Geometry: final body of the model. Coordinates: model frame, mm. A direction names the side the tool comes from. Round coordinates to 2 decimals unless told otherwise and drop trailing zeros. Loops run counter-clockwise (first coordinate to the right, second up) from the corner with the lowest first, then second, coordinate; pieces in that order, holes last. Notation, with made-up numbers: (0, -23.5) - (46, -23.5) arc R3 cw to (46, -18.5) - close; hole circle Ø9 at (61.25, -8.5). An arc over 180 degrees is marked (long way). Answer as a JSON object with one key per item and string values. Group by question number.
Item 1: Reachability of faces 1 (the face through (0, 0, -0.4)), 2 (the face through (4.91, 1.55, 0.74)) from +Z, -Z, +X, -X, +Y, -Y: full face, straight path, thin tool, end or side. Return the list, or none.
Item 2: First-contact query: pin 1 (2 mm diameter, centred on y = 2, z = 13, fed in from +X); pin 2 (10 mm diameter, centred on x = -5, y = -2, fed in from +Z); pin 3 (1 mm diameter, centred on y = -4, z = 12, fed in from -X). Flat tips, straight axial feed; report the tip coordinate or a pass-through.
Item 3: Section B-B (y = 11). Return the cut outline in (x, z), plus the area to 3 significant figures.
Item 4: Section A-A (x = 0). Return the cut outline in (y, z), plus the area to 3 significant figures.
Item 5: Section D-D (y = -0.5). Return the cut outline in (x, z), plus the area to 3 significant figures.
Item 6: Draft query along Y for faces 3 (the face through (-1.116, 5.972, 0.537)), 4 (the face through (5.4, -16.4, 16)). Return one class per face: released by +Y, released by -Y, zero draft, split by the parting line, or undercut.
Item 7: Line query: line 1 (Y direction, x = 0, z = 0.5); line 2 (Z direction, x = 8.5, y = 0); line 3 (X direction, y = -1, z = 13.25). Output: solid intervals per line, ascending.
Item 8: Section C-C (x = 9.5). Return the cut outline in (y, z), plus the area to 3 significant figures.
```python
from build123d import *

# Parameters (mm, degrees)
F2_R     = 18.5
F2_R_2   = 17
F2_R_3   = 5.15
F3_DEPTH = 0.4
F4_DEPTH = 1.5
F5_DEPTH = 16


with BuildPart() as f3:
    # F2 (on Top) → F3 (new body)
    with BuildSketch(Plane.XY):
        Circle(F2_R)
        Circle(F2_R_2, mode=Mode.SUBTRACT)
        Circle(F2_R_2)
        with Locations((0, -11)):
            Circle(F2_R_3, mode=Mode.SUBTRACT)
        Circle(F2_R_3, mode=Mode.SUBTRACT)
        with Locations((0, 11)):
            Circle(F2_R_3, mode=Mode.SUBTRACT)
        Circle(F2_R_3)
        with Locations((0, -11)):
            Circle(F2_R_3)
    extrude(amount=-F3_DEPTH)

    # F2 (on Top) → F4 (join)
    with BuildSketch(Plane.XY):
        Circle(F2_R_2)
        with Locations((0, -11)):
            Circle(F2_R_3, mode=Mode.SUBTRACT)
        Circle(F2_R_3, mode=Mode.SUBTRACT)
        with Locations((0, 11)):
            Circle(F2_R_3, mode=Mode.SUBTRACT)
    extrude(amount=F4_DEPTH)

    # F2 (on Top) → F5 (join)
    with BuildSketch(Plane.XY):
        Circle(F2_R)
        Circle(F2_R_2, mode=Mode.SUBTRACT)
    extrude(amount=F5_DEPTH)


solid = f3.part
```
Values:
{
 "1": {"face 1": "-Z, +X, -X, +Y, -Y", "face 2": "+Z"},
 "2": {"pin 1": "stops at x = 18.47", "pin 2": "stops at z = 1.5", "pin 3": "stops at x = -18.17"},
 "3": {"outline": "(-14.87, -0.4) - (-5.15, -0.4) - (-5.15, 1.5) - (-12.96, 1.5) - (-12.96, 16) - (-14.87, 16) - close; (5.15, -0.4) - (14.87, -0.4) - (14.87, 16) - (12.96, 16) - (12.96, 1.5) - (5.15, 1.5) - close", "area": "92.4 mm^2"},
 "4": {"outline": "(-18.5, -0.4) - (5.85, -0.4) - (5.85, 1.5) - (5.15, 1.5) - (5.15, 0) - (-5.15, 0) - (-5.15, 1.5) - (-5.85, 1.5) - (-5.85, 0) - (-16.15, 0) - (-16.15, 1.5) - (-17, 1.5) - (-17, 16) - (-18.5, 16) - close; (16.15, -0.4) - (18.5, -0.4) - (18.5, 16) - (17, 16) - (17, 1.5) - (16.15, 1.5) - close", "area": "63.3 mm^2"},
 "5": {"outline": "(-18.49, -0.4) - (18.49, -0.4) - (18.49, 16) - (16.99, 16) - (16.99, 1.5) - (5.13, 1.5) - (5.13, 0) - (-5.13, 0) - (-5.13, 1.5) - (-16.99, 1.5) - (-16.99, 16) - (-18.49, 16) - close", "area": "98.4 mm^2"},
 "6": {"face 3": "undercut", "face 4": "zero draft"},
 "7": {"line 1": "y = -18.5 to -16.15, -5.85 to -5.15, 5.15 to 5.85, 16.15 to 18.5", "line 2": "z = -0.4 to 1.5", "line 3": "x = -18.47 to -16.97, 16.97 to 18.47"},
 "8": {"outline": "(-15.87, -0.4) - (15.87, -0.4) - (15.87, 16) - (14.1, 16) - (14.1, 1.5) - (-14.1, 1.5) - (-14.1, 16) - (-15.87, 16) - close", "area": "112 mm^2"}
}
